Answer from the drawing. Dimensions are ordinates in mm from the lowest x, y and z of the part. Round coordinates to 2 decimals unless told otherwise and drop trailing zeros. Loops run counter-clockwise (first coordinate to the right, second up) from the corner with the lowest first, then second, coordinate; pieces in that order, holes last. Notation, with made-up numbers: (17.25, 17) - (28.25, 17) arc R17 ccw to (28.25, 40) - close; hole circle Ø11 at (-33, -26). An arc over 180 degrees is marked (long way). Answer as CSV lines item,"result". Start each with the question number.
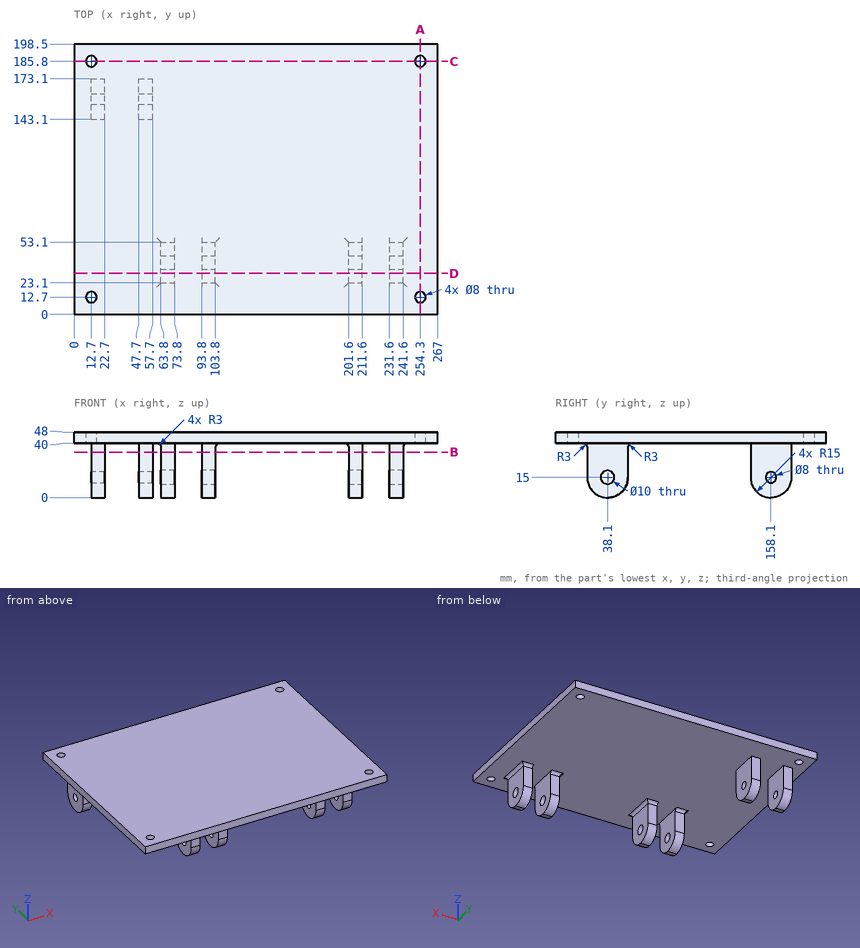
Item 1: Flat-ended cylindrical pins translate along their axes: pin 1 Ø3 at (x, z) = (235.5, 30.5) entering from +Y; pin 2 Ø8 at (x, y) = (192.5, 38) entering from -Z; pin 3 Ø5 at (x, z) = (67, 20.5) entering from -Y; pin 4 Ø8 at (y, z) = (38.1, 15) entering from -X. Find the tip coordinate at first contact, or state that the pin passes through.
Item 2: Section B-B, the plane z = 33.5 is taken. Give the vertices of the cut face in (x, y).
Item 3: Section A-A, the plane x = 254.3 is taken. Give the vertices of the cut face in (y, z).
Item 4: Section C-C, the plane y = 185.8 is taken. Give the vertices of the cut face in (x, z), and give its area (3 significant figures).
Item 5: Section D-D, the plane y = 30 is taken. Give the vertices of the cut face in (x, z) (3 decimals), and give its area (3 significant figures).
Item 6: Find the intervals of material crossed by L1, parallel to Y at x = 254.3, z = 45.25; L2, parallel to Z at x = 239, y = 38.1; L3, parallel to X at y = 164, z = 36.5, in increasing order.
Answer:
1,pin 1,"stops at y = 53.1"
1,pin 2,"stops at z = 40"
1,pin 3,"stops at y = 23.1"
1,pin 4,"passes through"
2,outline,"(12.7, 143.1) - (22.7, 143.1) - (22.7, 173.1) - (12.7, 173.1) - close; (47.7, 143.1) - (57.7, 143.1) - (57.7, 173.1) - (47.7, 173.1) - close; (63.8, 23.1) - (73.8, 23.1) - (73.8, 53.1) - (63.8, 53.1) - close; (93.8, 23.1) - (103.8, 23.1) - (103.8, 53.1) - (93.8, 53.1) - close; (201.6, 23.1) - (211.6, 23.1) - (211.6, 53.1) - (201.6, 53.1) - close; (231.6, 23.1) - (241.6, 23.1) - (241.6, 53.1) - (231.6, 53.1) - close"
3,outline,"(0, 40) - (8.7, 40) - (8.7, 48) - (0, 48) - close; (16.7, 40) - (181.8, 40) - (181.8, 48) - (16.7, 48) - close; (189.8, 40) - (198.5, 40) - (198.5, 48) - (189.8, 48) - close"
4,outline,"(0, 40) - (8.7, 40) - (8.7, 48) - (0, 48) - close; (16.7, 40) - (250.3, 40) - (250.3, 48) - (16.7, 48) - close; (258.3, 40) - (267, 40) - (267, 48) - (258.3, 48) - close"
4,area,"2,010 mm²"
5,outline,"(0, 40) - (60.8, 40) arc R3 cw to (63.8, 37) - (63.8, 2.375) - (73.8, 2.375) - (73.8, 40) - (93.8, 40) - (93.8, 2.375) - (103.8, 2.375) - (103.8, 37) arc R3 cw to (106.8, 40) - (198.6, 40) arc R3 cw to (201.6, 37) - (201.6, 2.375) - (211.6, 2.375) - (211.6, 40) - (231.6, 40) - (231.6, 2.375) - (241.6, 2.375) - (241.6, 37) arc R3 cw to (244.6, 40) - (267, 40) - (267, 48) - (0, 48) - close"
5,area,"3,650 mm²"
6,L1,"y = 0 to 8.7, 16.7 to 181.8, 189.8 to 198.5"
6,L2,"z = 0 to 10, 20 to 48"
6,L3,"x = 12.7 to 22.7, 47.7 to 57.7"
